Input: part model. Units: mm. Frame: model coordinates. A direction names the side the tool comes from. Coordinates: 2 decimals unless noted, no trailing zeros. Order: outer loops, then holes, each group sorted by start corner. A loop starts at its lowest first (then second) coordinate and runs counter-clockwise, first axis right, second up. Notation, with made-up numbers: (24, -28) - (53, -28) arc R24 cw to (53, 6) - close; hole circle Ø4 at (26, 9). An arc over 180 degrees is marked (long way). Use a Markdown table: item, result. Add a question column.
from build123d import *

# Parameters (mm, degrees)
ESQUISSE1_R        = 4
BOSS_EXTRU_1_DEPTH = 2
BOSS_EXTRU_2_DEPTH = 1.2


with BuildPart() as part:
    # Esquisse1 → Boss.-Extru.1 (new body)
    with BuildSketch(Plane.XY):
        with BuildLine():
            Line((-23.9, 14), (-14.282856857, 14))
            ThreePointArc((-14.282856857, 14), (0, 20), (14.282856857, 14))
            Line((14.282856857, 14), (23.9, 14))
            Line((23.9, 14), (23.9, 70))
            Line((23.9, 70), (6.965826107, 90.69888293))
            ThreePointArc((6.965826107, 90.69888293), (0, 94), (-6.965826107, 90.69888293))
            Line((-6.965826107, 90.69888293), (-23.9, 70))
            Line((-23.9, 70), (-23.9, 14))
        make_face()
        with Locations((0, 85)):
            Circle(ESQUISSE1_R, mode=Mode.SUBTRACT)
    extrude(amount=BOSS_EXTRU_1_DEPTH)

    # Esquisse2 → Boss.-Extru.2 (add)
    with BuildSketch(Plane.XY.offset(2)):
        Polygon((-23.9, 14), (-20.9, 14), (-20.9, 73.666942904), (-23.9, 70), align=None)
        Polygon((23.9, 14), (20.9, 14), (20.9, 73.666942904), (23.9, 70), align=None)
    extrude(amount=BOSS_EXTRU_2_DEPTH)


solid = part.part
1) Cut plane D-D (y = 85). Return the cut outline in (x, z).
2) Contact query for flat-ended pins moving along their axis: P1, Ø4, axis at x = -9.5, y = 82, coming from the -Z side; P2, Ø1.5, axis at x = 10.5, y = 42, coming from the +Z side. Output: stop coordinate, or through.
3) Cut plane A-A (x = 0). Return the cut outline in (y, z), and give its area (3 significant figures).
4) Cut plane C-C (y = 34.5). Return the cut outline in (x, z).
5) Cut plane B-B (z = 0.5). Return the cut outline in (x, y), and give its area (3 significant figures).
6) Material intervals for L1, parallel to X at y = 35.5, z = 2.55; L2, parallel to Z at x = -19, y = 43; L3, parallel to X at y = 82, z = 1.1, sorted ascending.
7) Reachability of faces 1 (the flat face through (0, 55, 0)), 2 (the flat face through (0, 55, 2)) from +Z, -Z, +X, -X, +Y, -Y: full face, straight path, thin tool, end or side. Return the list, or none.
8) Pull-direction query (X, two-part tool) for faces 3 (the cylindrical face through (0, 20, 1)), 4 (the flat face through (-23.9, 42, 2)), 5 (the flat face through (23.9, 42, 2)), 6 (the flat face through (22, 44, 3.2)); classes: pulls with the +X half, pulls with the -X half, needs draft (parallel to the pull), parting line crosses it, or undercut.
Computed:
| question | item | result |
|---|---|---|
| 1 | outline | (-11.63, 0) - (-4, 0) - (-4, 2) - (-11.63, 2) - close; (4, 0) - (11.63, 0) - (11.63, 2) - (4, 2) - close |
| 2 | P1 | stops at z = 0 |
| 2 | P2 | stops at z = 2 |
| 3 | outline | (20, 0) - (81, 0) - (81, 2) - (20, 2) - close; (89, 0) - (94, 0) - (94, 2) - (89, 2) - close |
| 3 | area | 132 mm2 |
| 4 | outline | (-23.9, 0) - (23.9, 0) - (23.9, 3.2) - (20.9, 3.2) - (20.9, 2) - (-20.9, 2) - (-20.9, 3.2) - (-23.9, 3.2) - close |
| 5 | outline | (-23.9, 14) - (-14.28, 14) arc R20 cw to (14.28, 14) - (23.9, 14) - (23.9, 70) - (6.97, 90.7) arc R9 ccw to (-6.97, 90.7) - (-23.9, 70) - close; hole circle Ø8 at (0, 85) |
| 5 | area | 3,180 mm2 |
| 6 | L1 | x = -23.9 to -20.9, 20.9 to 23.9 |
| 6 | L2 | z = 0 to 2 |
| 6 | L3 | x = -14.08 to -2.65, 2.65 to 14.08 |
| 7 | face 1 | -Z, +X, -X, +Y, -Y |
| 7 | face 2 | +Z, +Y, -Y |
| 8 | face 3 | undercut |
| 8 | face 4 | pulls with the -X half |
| 8 | face 5 | pulls with the +X half |
| 8 | face 6 | needs draft |
